```python
from build123d import *

# Parameters (mm, degrees)
SKETCH1_R           = 2.9718
BOSS_EXTRUDE1_DEPTH = 2.54


with BuildPart() as part:
    # Sketch1 → Boss-Extrude1 (new body)
    with BuildSketch(Plane.XY):
        with BuildLine():
            Line((-46.99, 10.16), (0, 10.16))
            Line((0, 10.16), (5.08, 10.16))
            ThreePointArc((5.08, 10.16), (8.672102448, 8.672102448), (10.16, 5.08))
            Line((10.16, 5.08), (10.16, 0))
            Line((10.16, 0), (10.16, -5.08))
            ThreePointArc((10.16, -5.08), (8.672102448, -8.672102448), (5.08, -10.16))
            Line((5.08, -10.16), (-46.99, -10.16))
            Line((-46.99, -10.16), (-52.07, -10.16))
            ThreePointArc((-52.07, -10.16), (-55.662102448, -8.672102448), (-57.15, -5.08))
            Line((-57.15, -5.08), (-57.15, 5.08))
            ThreePointArc((-57.15, 5.08), (-55.662102448, 8.672102448), (-52.07, 10.16))
            Line((-52.07, 10.16), (-46.99, 10.16))
        make_face()
        Circle(SKETCH1_R, mode=Mode.SUBTRACT)
        with Locations((-46.99, 0)):
            Circle(SKETCH1_R, mode=Mode.SUBTRACT)
    extrude(amount=BOSS_EXTRUDE1_DEPTH)


solid = part.part
```
Read the model definition and answer for the solid it produces. Units are mm, in the model's axes. Coordinates: 2 decimals unless noted, no trailing zeros. Write each loop counter-clockwise with the first axis right and the second up, starting at its lowest first coordinate (ties: lowest second). Pieces come first, ordered by that corner, then holes. Notation, with made-up numbers: (85, 11.25) - (127, 11.25) arc R24 ccw to (127, 34.25) - close; hole circle Ø10 at (6.5, -14). An arc over 180 degrees is marked (long way). Answer as a JSON object with one key per item and string values. Group by question number.
1. This flat-tipped pin is pushed along its axis until it touches: P1, Ø5, axis at x = -46.99, y = 0, coming from the +Z side. Where does it stop, or does it pass through?
2. A cutting plane is placed at A-A (z = 1.85). Determine the outline of the cut face in (x, y).
3. A cutting plane is placed at B-B (y = 0). Determine the outline of the cut face in (x, z).
4. A cutting plane is placed at C-C (x = -46.99). Determine the outline of the cut face in (y, z).
5. A cutting plane is placed at D-D (y = -7.75). Determine the outline of the cut face in (x, z).
6. Consider L1, parallel to X at y = -0.25, z = 2.3; L2, parallel to X at y = 1, z = 0.65; L3, parallel to Y at x = -46.99, z = 1.5. Determine where each line is inside the solid, lowest interval first. Write a range as [from, to].
7. The mould has two halves that part along X. Classify faces 1 (the flat face through (-24, 10.16, 1)), 2 (the cylindrical face through (2.835, 0.893, 1.252)), 3 (the flat face through (10.16, 0, 1)): +X half, -X half, draft (parallel to the pull), parting line (faces both ways), or undercut.
Worked out:
{
 "1": {"P1": "passes through"},
 "2": {"outline": "(-57.15, -5.08) arc R5.08 ccw to (-52.07, -10.16) - (5.08, -10.16) arc R5.08 ccw to (10.16, -5.08) - (10.16, 5.08) arc R5.08 ccw to (5.08, 10.16) - (-52.07, 10.16) arc R5.08 ccw to (-57.15, 5.08) - close; hole circle Ø5.94 at (-46.99, 0); hole circle Ø5.94 at (0, 0)"},
 "3": {"outline": "(-57.15, 0) - (-49.96, 0) - (-49.96, 2.54) - (-57.15, 2.54) - close; (-44.02, 0) - (-2.97, 0) - (-2.97, 2.54) - (-44.02, 2.54) - close; (2.97, 0) - (10.16, 0) - (10.16, 2.54) - (2.97, 2.54) - close"},
 "4": {"outline": "(-10.16, 0) - (-2.97, 0) - (-2.97, 2.54) - (-10.16, 2.54) - close; (2.97, 0) - (10.16, 0) - (10.16, 2.54) - (2.97, 2.54) - close"},
 "5": {"outline": "(-56.39, 0) - (9.4, 0) - (9.4, 2.54) - (-56.39, 2.54) - close"},
 "6": {"L1": "x = [-57.15, -49.95], [-44.03, -2.96], [2.96, 10.16]", "L2": "x = [-57.15, -49.79], [-44.19, -2.8], [2.8, 10.16]", "L3": "y = [-10.16, -2.97], [2.97, 10.16]"},
 "7": {"face 1": "draft", "face 2": "undercut", "face 3": "+X half"}
}
